from build123d import *

# Parameters (mm, degrees)
F1_DEPTH = 6.35
F2_R     = 5.08


with BuildPart() as f1:
    # F0 (on Front) → F1 (new body)
    with BuildSketch(Plane.XZ):
        with BuildLine():
            ThreePointArc((-25.1582770203, -3.4958686142), (-17.6652781796, -18.2509711204), (-2.6737065925, -25.2588854279))
            ThreePointArc((-2.6737065925, -25.2588854279), (-3.505224173, -13.0246794199), (2.277990057, -2.2116478698))
            ThreePointArc((2.277990057, -2.2116478698), (-2.2081596575, -2.2813715013), (-2.2847476043, 2.2046662752))
            ThreePointArc((-2.2847476043, 2.2046662752), (-12.90346397, -3.9280392538), (-25.1582770203, -3.4958686142))
        make_face()
        with BuildLine():
            ThreePointArc((-2.2847476043, 2.2046662752), (-2.2081596575, -2.2813715013), (2.277990057, -2.2116478698))
            ThreePointArc((2.277990057, -2.2116478698), (2.942213744, -1.1933160874), (3.175, 0))
            ThreePointArc((3.175, 0), (2.9440362131, 1.1888127589), (2.2847475428, 2.2046663389))
            ThreePointArc((2.2847475428, 2.2046663389), (-4.43e-08, 3.175), (-2.2847476043, 2.2046662752))
        make_face()
    extrude(amount=F1_DEPTH)

    # F2
    f2_edges = [f1.edges().sort_by_distance(p)[0] for p in [
        (-17.665278, -6.35, -18.250971),
    ]]
    fillet(f2_edges, radius=F2_R)


solid = f1.part
Can you work these out from the model? Positions are in its coordinate system, mm. Give positions to 0.01 mm unless a question says otherwise; leave off trailing zeros. Loops run counter-clockwise (first coordinate to the right, second up) from the corner with the lowest first, then second, coordinate; pieces in that order, holes last. Notation, with made-up numbers: M -13,-3 L 40,-3 A30 cw 40,34 Z; hole C 18.25,-30.75 d11. An arc over 180 degrees is marked long. One line per item, written item: value. Start each with the question number.
1) Thinking about a two-plate mould opening in X: for faces 1 (the face through (-11, 0, -11)), 2 (the face through (-12.735, -3.131, -3.885)), 3 (the face through (-17.83, -0.63, -18.09)), which applies, +X half, -X half, draft (parallel to the pull), parting line (faces both ways), or undercut?
2) If we section it at B-B, the plane x = 0.5: Write out the boundary of the cut face in (y, z), and give its area (3 significant figures).
3) If we section it at A-A, the plane y = -2.25: Write out the boundary of the cut face in (x, z) (3 decimals).
4) If I drill on line 1 (Z direction, x = -22.5, y = -0.5); line 2 (Z direction, x = -12.75, y = -5.75); line 3 (X direction, y = -0.5, z = -6.75), over which ranges is the centre line in solid material (lowest first)? Write a range as [from, to].
5) I'm going to push a flat-ended pin straight in: pin 1 (6 mm diameter, centred on x = -3.5, z = -15, fed in from +Y). Where does the tip first touch, or does it pass through?
6) If we section it at C-C, the plane y = -5.5: Write out the boundary of the cut face in (x, z) (3 decimals).
Completed:
1. face 1: draft
1. face 2: undercut
1. face 3: -X half
2. outline: M -6.35,-4.28 L 0,-4.28 L 0,3.14 L -6.35,3.14 Z
2. area: 47.1 mm^2
3. outline: M -25.057,-3.528 A25.305 ccw -2.71,-25.159 A22.225 cw 2.278,-2.212 A3.175 ccw -2.285,2.205 A22.225 cw Z
4. line 1: z = [-11.79, -4.18]
4. line 2: z = [-18.8, -3.89]
4. line 3: x = [-24.49, -1.12]
5. pin 1: stops at y = 0
6. outline: M -22.761,-4.131 A23.133 ccw -3.386,-22.884 A22.225 cw 2.278,-2.212 A3.175 ccw -2.285,2.205 A22.225 cw Z
